Check sheet for the modelled part. Datum: model origin and axes. Units: mm. A direction names the side the tool comes from. Give positions to 0.01 mm unless a question says otherwise; leave off trailing zeros. Loops run counter-clockwise (first coordinate to the right, second up) from the corner with the lowest first, then second, coordinate; pieces in that order, holes last.
```python
from build123d import *

# Parameters (mm, degrees)
SKETCH1_W           = 4
SKETCH1_H           = 15
BOSS_EXTRUDE1_DEPTH = 4


with BuildPart() as part:
    # Sketch1 → Boss-Extrude1 (new body)
    with BuildSketch(Plane.XY):
        Polygon((-75, -50), (75, -50), (110, -50), (110, 50), (75, 50), (-75, 50), align=None)
        with BuildLine():
            Line((-46.516283173, 20), (43.374974686, 20))
            ThreePointArc((43.374974686, 20), (-1.570654243, -32.179711562), (-46.516283173, 20))
        make_face(mode=Mode.SUBTRACT)
        with Locations((58, 27.5)):
            Rectangle(SKETCH1_W, SKETCH1_H, mode=Mode.SUBTRACT)
        with Locations((58, -27.5)):
            Rectangle(SKETCH1_W, SKETCH1_H, mode=Mode.SUBTRACT)
        with Locations((-58, -27.5)):
            Rectangle(SKETCH1_W, SKETCH1_H, mode=Mode.SUBTRACT)
        with Locations((-58, 27.5)):
            Rectangle(SKETCH1_W, SKETCH1_H, mode=Mode.SUBTRACT)
        with Locations((103, 27.5)):
            Rectangle(SKETCH1_W, SKETCH1_H, mode=Mode.SUBTRACT)
        with Locations((103, -27.5)):
            Rectangle(SKETCH1_W, SKETCH1_H, mode=Mode.SUBTRACT)
    extrude(amount=BOSS_EXTRUDE1_DEPTH)


solid = part.part
```
(1) Access from +Z, -Z, +X, -X, +Y, -Y to the whole of each face (thin tool, end or side, straight path). Record for faces 5 (the face through (16, -50, 2)), 6 (the face through (-2, 20, 2)).
(2) Material ranges on line 1 (X direction, y = 24, z = 1.15); line 2 (Y direction, x = -0.5, z = 3.6); line 3 (X direction, y = 12, z = 0.7), recorded low to high.
(3) Release check for a two-part mould opening along X. For faces 1 (the face through (16, 23, 4)), 2 (the face through (56, -28, 2)), 3 (the face through (110, -1, 2)), 4 (the face through (-0.477, -32.167, 1.972)) record: pulls with the +X half, pulls with the -X half, needs draft (parallel to the pull), parting line crosses it, or undercut.
(4) Section check A-A on y = 25. Record the boundary of the cut face in (x, z).
(5) Section check B-B on x = -24. Record the boundary of the cut face in (y, z).
(6) Section check D-D on y = -25. Record the boundary of the cut face in (x, z), plus the area to 3 significant figures.
(7) Section check C-C on z = 2.6. Give the number of separate pieces and of enclosed holes in the cut face, plus the area to 3 significant figures.
Computed values:
1. face 5: +Z, -Z, +X, -X, -Y
1. face 6: +Z, -Z
2. line 1: x = -75 to -60, -56 to 56, 60 to 101, 105 to 110
2. line 2: y = -50 to -32.17, 20 to 50
2. line 3: x = -75 to -47, 43.86 to 110
3. face 1: needs draft
3. face 2: undercut
3. face 3: pulls with the +X half
3. face 4: undercut
4. outline: (-75, 0) - (-60, 0) - (-60, 4) - (-75, 4) - close; (-56, 0) - (56, 0) - (56, 4) - (-56, 4) - close; (60, 0) - (101, 0) - (101, 4) - (60, 4) - close; (105, 0) - (110, 0) - (110, 4) - (105, 4) - close
5. outline: (-50, 0) - (-26.26, 0) - (-26.26, 4) - (-50, 4) - close; (20, 0) - (50, 0) - (50, 4) - (20, 4) - close
6. outline: (-75, 0) - (-60, 0) - (-60, 4) - (-75, 4) - close; (-56, 0) - (-26.09, 0) - (-26.09, 4) - (-56, 4) - close; (22.95, 0) - (56, 0) - (56, 4) - (22.95, 4) - close; (60, 0) - (101, 0) - (101, 4) - (60, 4) - close; (105, 0) - (110, 0) - (110, 4) - (105, 4) - close
6. area: 496 mm2
7. separate pieces: 1
7. enclosed holes: 7
7. area: 14,300 mm2
